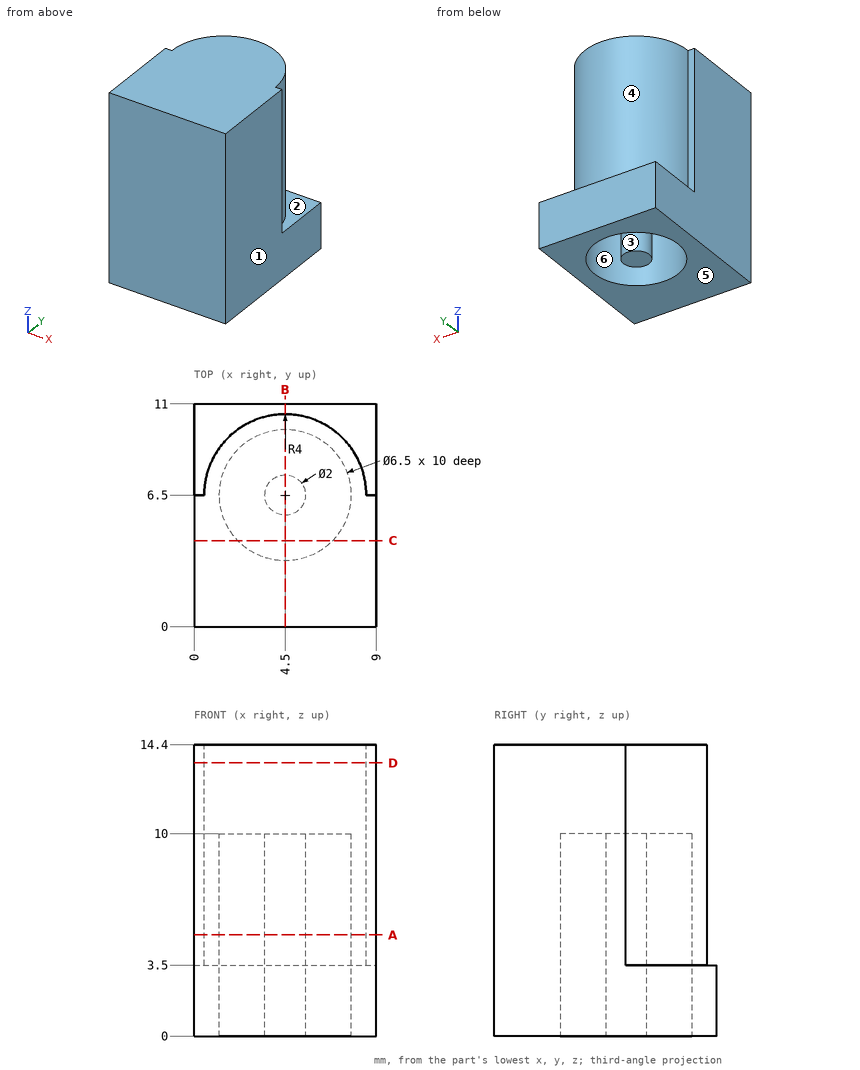
Design review of the part shown in the three views and the two pictorial views. Dimensions are in mm from the part's minimum x, y and z. A direction names the side the tool comes from. Round coordinates to 2 decimals unless told otherwise and drop trailing zeros. Write each loop counter-clockwise with the first axis right and the second up, starting at its lowest first coordinate (ties: lowest second). Pieces come first, ordered by that corner, then holes. Notation, with made-up numbers: (46, 36) -> (55, 36) arc R5 ccw to (55, 43) -> close; hole circle Ø9 at (15, 83). An arc over 180 degrees is marked (long way). Use one line per item in the form item = value.
1) Take a section at B-B, the plane x = 4.5. Write out the cut boundary in (y, z), and give its area (3 significant figures).
Found:
outline = (0, 0) -> (3.25, 0) -> (3.25, 10) -> (5.5, 10) -> (5.5, 0) -> (7.5, 0) -> (7.5, 10) -> (9.75, 10) -> (9.75, 0) -> (11, 0) -> (11, 3.5) -> (10.5, 3.5) -> (10.5, 14.4) -> (0, 14.4) -> close
area = 108 mm2
2) Take a section at C-C, the plane y = 4.25. Write out the cut boundary in (x, z), and give its area (3 significant figures).
Found:
outline = (0, 0) -> (2.15, 0) -> (2.15, 10) -> (6.85, 10) -> (6.85, 0) -> (9, 0) -> (9, 14.4) -> (0, 14.4) -> close
area = 82.7 mm2
3) To check wall thickness, follow L1, parallel to Y at x = 4.5, z = 3; L2, parallel to Y at x = 4.5, z = 6.75; L3, parallel to X at y = 6, z = 7.75. State the ranges of each line that lie inside material, in increasing order. Write a range as from..to.
Found:
L1 = 0..3.25, 5.5..7.5, 9.75..11
L2 = 0..3.25, 5.5..7.5, 9.75..10.5
L3 = 0..1.29, 3.63..5.37, 7.71..9
4) Take a section at D-D, the plane z = 13.5. Write out the cut boundary in (x, y), and give its area (3 significant figures).
Found:
outline = (0, 0) -> (9, 0) -> (9, 6.5) -> (8.5, 6.5) arc R4 ccw to (0.5, 6.5) -> (0, 6.5) -> close
area = 83.6 mm2
5) Tool access review of the marked faces 5 and 6: name each direction out of +Z, -Z, +X, -X, +Y, -Y from which nothing blocks a thin tool from reaching the whole face with its end or side.
Found:
face_5 = -Z, +X, -X, +Y, -Y
face_6 = -Z
6) Mouldability with a two-part tool opening along X and no side actions: class the marked faces 1, 2, 3 and 4 as +X half, -X half, draft (parallel to the pull), parting line (faces both ways), or undercut.
Found:
face_1 = +X half
face_2 = draft
face_3 = undercut
face_4 = parting line
7) Take a section at A-A, the plane z = 5. Write out the cut boundary in (x, y).
Found:
outline = (0, 0) -> (9, 0) -> (9, 6.5) -> (8.5, 6.5) arc R4 ccw to (0.5, 6.5) -> (0, 6.5) -> close; circle Ø2 at (4.5, 6.5); hole circle Ø6.5 at (4.5, 6.5)
